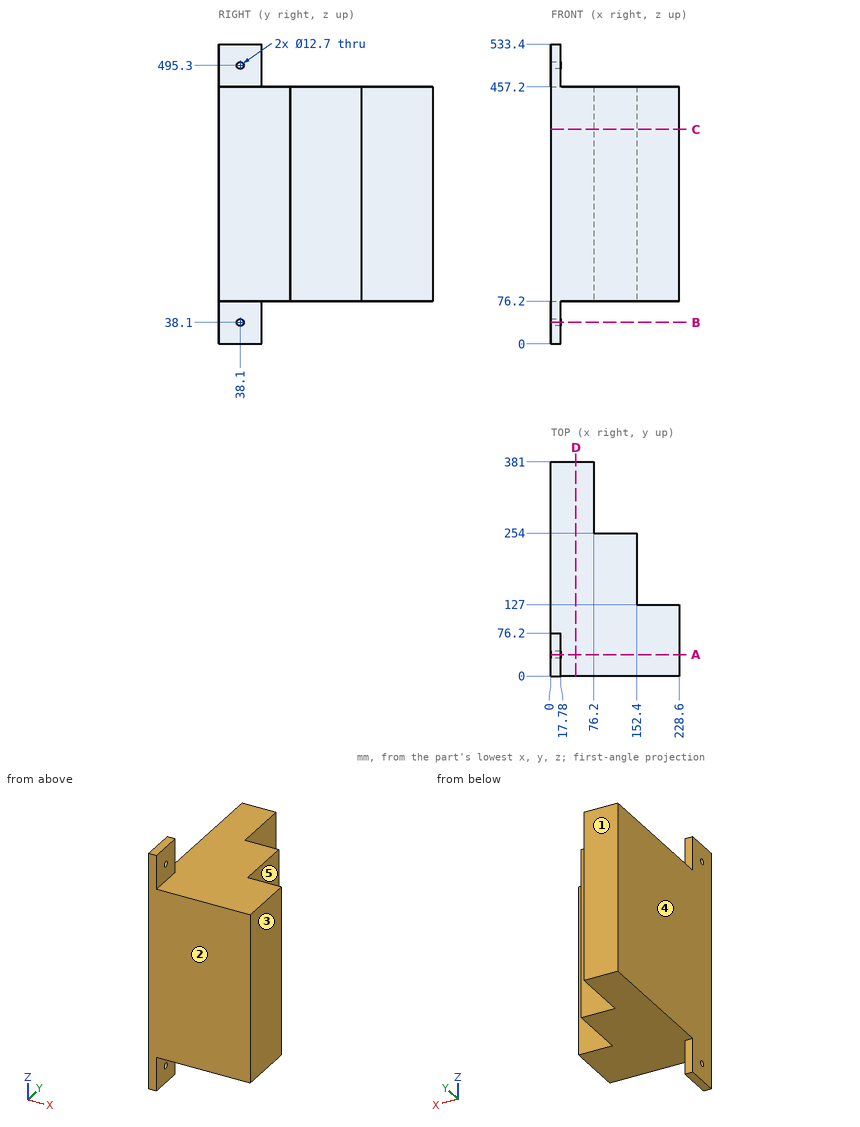
Geometry: see drawing. Coordinates: mm, zero at the bounding-box minimum. A direction names the side the tool comes from. Give positions to 0.01 mm unless a question says otherwise; leave off trailing zeros. Order: outer loops, then holes, each group sorted by start corner. A loop starts at its lowest first (then second) coordinate and runs counter-clockwise, first axis right, second up. Notation, with made-up numbers: M 72.5,74 L 107.5,74 A22 ccw 107.5,87 Z; hole C 66.5,2.25 d1. An arc over 180 degrees is marked long. Answer as CSV lines item,"result". Start each with the question number.
1) Cut plane B-B (z = 38.1). Output: boundary loops of the cut face in (x, y).
2) Cut plane C-C (z = 381.5). Output: boundary loops of the cut face in (x, y), then the cut area to 3 significant figures.
3) Set-up query: the marked faces 4 and 5. Return all of +Z, -Z, +X, -X, +Y, -Y with unobstructed straight access to the full face (end or side cutting, diameter ignored); none if empty.
4) Mould query, pull axis Y, two halves, no side actions, for the marked faces 1, 2 and 3. Classes: +Y half, -Y half, draft (parallel to the pull), parting line (faces both ways), or undercut.
5) Cut plane A-A (y = 38.1). Output: boundary loops of the cut face in (x, z).
6) Cut plane D-D (x = 44.5). Output: boundary loops of the cut face in (y, z).
7) First-contact query: P1, Ø1, axis at y = 275, z = 405, coming from the +X side; P2, Ø1, axis at y = 76, z = 178.5, coming from the -X side; P3, Ø5.5, axis at x = 11.5, z = 489, coming from the +Y side; P4, Ø23, axis at x = 125, z = 186, coming from the +Y side. Flat tips, straight axial feed; report the tip coordinate or a pass-through.
8) Line query: line 1 (Z direction, x = 8, y = 38); line 2 (Y direction, x = 4, z = 495); line 3 (Z direction, x = 16, y = 158.5). Output: solid intervals per line, ascending. Write a range as from..to.
Findings below:
1,outline,"M 0,0 L 17.78,0 L 17.78,31.75 L 0,31.75 Z; M 0,44.45 L 17.78,44.45 L 17.78,76.2 L 0,76.2 Z"
2,outline,"M 0,0 L 228.6,0 L 228.6,127 L 152.4,127 L 152.4,254 L 76.2,254 L 76.2,381 L 0,381 Z"
2,area,"58,100 mm²"
3,face 4,"+Z, -Z, -X, +Y, -Y"
3,face 5,"+Z, -Z, +X, +Y"
4,face 1,"+Y half"
4,face 2,"-Y half"
4,face 3,"draft"
5,outline,"M 0,0 L 17.78,0 L 17.78,31.75 L 0,31.75 Z; M 0,44.45 L 17.78,44.45 L 17.78,76.2 L 228.6,76.2 L 228.6,457.2 L 17.78,457.2 L 17.78,488.95 L 0,488.95 Z; M 0,501.65 L 17.78,501.65 L 17.78,533.4 L 0,533.4 Z"
6,outline,"M 0,76.2 L 381,76.2 L 381,457.2 L 0,457.2 Z"
7,P1,"stops at x = 76.2"
7,P2,"stops at x = 0"
7,P3,"stops at y = 76.2"
7,P4,"stops at y = 254"
8,line 1,"z = 0..31.75, 44.45..488.95, 501.65..533.4"
8,line 2,"y = 0..31.76, 44.44..76.2"
8,line 3,"z = 76.2..457.2"
